Can you work these out from the model? Positions are in its coordinate system, mm. Face numbers are marked on the shaded views. Coordinates: 2 decimals unless noted, no trailing zeros. Loops run counter-clockwise (first coordinate to the right, second up) from the corner with the lowest first, then second, coordinate; pieces in that order, holes last.
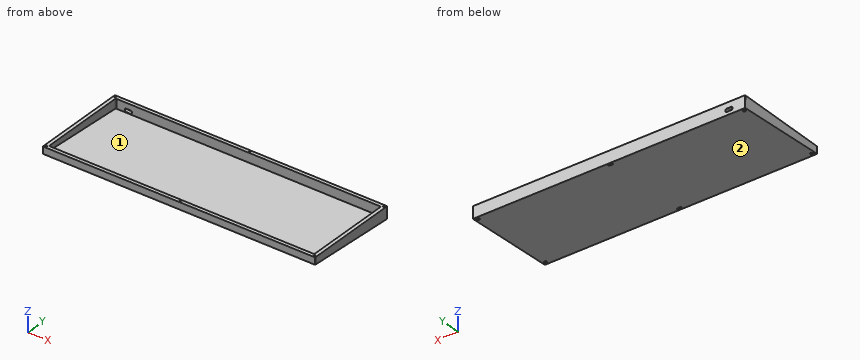
```python
from build123d import *

# Parameters (mm, degrees)
SKETCH3_W               = 431.8
SKETCH3_H               = 150.876
BOSS_EXTRUDE2_DEPTH     = 19.05
CUT_EXTRUDE4_DEPTH      = 432.8
SKETCH3_25_W            = 197.6453584
SKETCH3_25_H            = 139.766716802
SKETCH3_25_W_2          = 25.4
SKETCH3_25_W_3          = 197.645358401
CUT_EXTRUDE5_DEPTH      = 20.05
CUT_EXTRUDE5_DEPTH_BACK = 1
BOSS_EXTRUDE3_REACH     = 433.8
M2_CLEARANCE_HOLE1_D    = 2.4
CUT_EXTRUDE8_DEPTH      = 10.16
CUT_EXTRUDE9_DEPTH      = 2.032
FILLET7_R               = 1.5875
FILLET8_R               = 0.508
CUT_EXTRUDE10_REACH     = 152.876


with BuildPart() as part:
    # Sketch3 → Boss-Extrude2 (new body)
    with BuildSketch(Plane.XY):
        with Locations((169.861119801, 72.517452108)):
            Rectangle(SKETCH3_W, SKETCH3_H)
    extrude(amount=BOSS_EXTRUDE2_DEPTH)

    # Sketch11 → Cut-Extrude4 (cut, through all)
    with BuildSketch(Plane.ZY.offset(46.038880199)):
        Polygon((7.907076107, -2.920547892), (0, 147.955452108), (0, -2.920547892), align=None)
    extrude(amount=-CUT_EXTRUDE4_DEPTH, mode=Mode.SUBTRACT)

    # Sketch3<25> → Cut-Extrude5 (cut, two sides)
    with BuildSketch(Plane.XY) as cut_extrude5_sk:
        with Locations((281.383799001, 72.517452108)):
            Rectangle(SKETCH3_25_W, SKETCH3_25_H)
        with Locations((169.861119801, 72.517452108)):
            Rectangle(SKETCH3_25_W_2, SKETCH3_25_H)
        with Locations((58.338440601, 72.517452108)):
            Rectangle(SKETCH3_25_W_3, SKETCH3_25_H)
        with BuildLine():
            Line((-38.844861429, 142.400810509), (-40.4842386, 142.400810509))
            Line((-40.4842386, 142.400810509), (-40.4842386, 140.761433338))
            ThreePointArc((-40.4842386, 140.761433338), (-39.407803363, 141.324375272), (-38.844861429, 142.400810509))
        make_face()
        with BuildLine():
            ThreePointArc((-38.844861429, 2.634093707), (-39.407803363, 3.710528944), (-40.4842386, 4.273470879))
            Line((-40.4842386, 4.273470879), (-40.4842386, 2.634093707))
            Line((-40.4842386, 2.634093707), (-38.844861429, 2.634093707))
        make_face()
        with BuildLine():
            ThreePointArc((380.206478201, 4.273470879), (379.130042964, 3.710528944), (378.56710103, 2.634093707))
            Line((378.56710103, 2.634093707), (380.206478201, 2.634093707))
            Line((380.206478201, 2.634093707), (380.206478201, 4.273470879))
        make_face()
        with BuildLine():
            Line((380.206478201, 142.400810509), (378.56710103, 142.400810509))
            ThreePointArc((378.56710103, 142.400810509), (379.130042964, 141.324375272), (380.206478201, 140.761433338))
            Line((380.206478201, 140.761433338), (380.206478201, 142.400810509))
        make_face()
    extrude(amount=CUT_EXTRUDE5_DEPTH, mode=Mode.SUBTRACT)
    extrude(cut_extrude5_sk.sketch, amount=-CUT_EXTRUDE5_DEPTH_BACK, mode=Mode.SUBTRACT)

    # Sketch11<3> → Boss-Extrude3 (add, up to next)
    with BuildSketch(Plane.ZY.offset(46.038880199), mode=Mode.PRIVATE) as boss_extrude3_sk1:
        Polygon((3.815228638, 147.955452108), (0, 147.955452108), (7.907076107, -2.920547892), (11.722304745, -2.920547892), align=None)
    boss_extrude3_tool1 = extrude(boss_extrude3_sk1.sketch, amount=-BOSS_EXTRUDE3_REACH, mode=Mode.PRIVATE) - part.part
    add(boss_extrude3_tool1.solids().sort_by_distance((-46.03888, 72.517452, 5.861152))[0])

    # M2 Clearance Hole1 (through all)
    with Locations(Plane.XY.offset(19.05)):
        with Locations((-42.863880199, 144.780452108), (169.861119801, 144.780452108), (382.586119801, 144.780452108), (382.586119801, 0.254452108), (169.861119801, 0.254452108), (-42.863880199, 0.254452108)):
            Hole(M2_CLEARANCE_HOLE1_D / 2)

    # Sketch3<27> → Cut-Extrude8 (cut)
    with BuildSketch(Plane.XY):
        with BuildLine():
            Line((-44.795957036, 1.196057231), (-42.281485322, 3.710528944))
            ThreePointArc((-42.281485322, 3.710528944), (-39.407803363, 3.710528944), (-39.407803363, 0.836846986))
            Line((-39.407803363, 0.836846986), (-41.922275077, -1.677624728))
            ThreePointArc((-41.922275077, -1.677624728), (-44.795957036, -1.677624728), (-44.795957036, 1.196057231))
        make_face()
        with BuildLine():
            Line((168.083119801, 2.286452108), (171.639119801, 2.286452108))
            ThreePointArc((171.639119801, 2.286452108), (173.671119801, 0.254452108), (171.639119801, -1.777547892))
            Line((171.639119801, -1.777547892), (168.083119801, -1.777547892))
            ThreePointArc((168.083119801, -1.777547892), (166.051119801, 0.254452108), (168.083119801, 2.286452108))
        make_face()
        with BuildLine():
            Line((382.003724923, 3.710528944), (384.518196637, 1.196057231))
            ThreePointArc((384.518196637, 1.196057231), (384.518196637, -1.677624728), (381.644514678, -1.677624728))
            Line((381.644514678, -1.677624728), (379.130042964, 0.836846986))
            ThreePointArc((379.130042964, 0.836846986), (379.130042964, 3.710528944), (382.003724923, 3.710528944))
        make_face()
    extrude(amount=CUT_EXTRUDE8_DEPTH, mode=Mode.SUBTRACT)

    # Sketch3<28> → Cut-Extrude9 (cut)
    with BuildSketch(Plane.XY):
        with BuildLine():
            Line((168.083119801, 142.748452108), (171.639119801, 142.748452108))
            ThreePointArc((171.639119801, 142.748452108), (173.671119801, 144.780452108), (171.639119801, 146.812452108))
            Line((171.639119801, 146.812452108), (168.083119801, 146.812452108))
            ThreePointArc((168.083119801, 146.812452108), (166.051119801, 144.780452108), (168.083119801, 142.748452108))
        make_face()
        with BuildLine():
            Line((379.130042964, 144.198057231), (381.644514678, 146.712528944))
            ThreePointArc((381.644514678, 146.712528944), (384.518196637, 146.712528944), (384.518196637, 143.838846986))
            Line((384.518196637, 143.838846986), (382.003724923, 141.324375272))
            ThreePointArc((382.003724923, 141.324375272), (379.130042964, 141.324375272), (379.130042964, 144.198057231))
        make_face()
        with BuildLine():
            Line((-44.795957036, 143.838846986), (-42.281485322, 141.324375272))
            ThreePointArc((-42.281485322, 141.324375272), (-39.407803363, 141.324375272), (-39.407803363, 144.198057231))
            Line((-39.407803363, 144.198057231), (-41.922275077, 146.712528944))
            ThreePointArc((-41.922275077, 146.712528944), (-44.795957036, 146.712528944), (-44.795957036, 143.838846986))
        make_face()
    extrude(amount=CUT_EXTRUDE9_DEPTH, mode=Mode.SUBTRACT)

    # Fillet7
    fillet7_edges = [part.edges().sort_by_distance(p)[0] for p in [
        (380.206478201, 2.634093707, 15.240599157),
        (380.206478201, 142.400810509, 11.578167535),
        (-40.4842386, 142.400810509, 11.578167535),
        (-40.4842386, 2.634093707, 15.240599157),
    ]]
    fillet(fillet7_edges, radius=FILLET7_R)

    # Fillet8
    fillet8_edges = [part.edges().sort_by_distance(p)[0] for p in [
        (385.761119801, 147.955452108, 9.525),
        (-46.038880199, 147.955452108, 9.525),
        (-46.038880199, -2.920547892, 13.478538054),
        (385.761119801, -2.920547892, 13.478538054),
    ]]
    fillet(fillet8_edges, radius=FILLET8_R)

    # Sketch18 → Cut-Extrude10 (cut, up to next)
    with BuildSketch(Plane(origin=(0, 147.955452108, 0), x_dir=(1, 0, 0), z_dir=(0, 1, 0)), mode=Mode.PRIVATE) as cut_extrude10_sk1:
        with BuildLine():
            Line((-16.828880199, -10.16), (-23.940880199, -10.16))
            ThreePointArc((-23.940880199, -10.16), (-25.287918618, -9.602038418), (-25.845880199, -8.255))
            Line((-25.845880199, -8.255), (-25.845880199, -6.985))
            ThreePointArc((-25.845880199, -6.985), (-25.287918618, -5.637961582), (-23.940880199, -5.08))
            Line((-23.940880199, -5.08), (-16.828880199, -5.08))
            ThreePointArc((-16.828880199, -5.08), (-15.481841781, -5.637961582), (-14.923880199, -6.985))
            Line((-14.923880199, -6.985), (-14.923880199, -8.255))
            ThreePointArc((-14.923880199, -8.255), (-15.481841781, -9.602038418), (-16.828880199, -10.16))
        make_face()
    cut_extrude10_tool1 = extrude(cut_extrude10_sk1.sketch, amount=-CUT_EXTRUDE10_REACH, mode=Mode.PRIVATE) & part.part
    add(cut_extrude10_tool1.solids().sort_by_distance((-20.38488, 147.955452, 7.62))[0], mode=Mode.SUBTRACT)


solid = part.part
```
(1) If I drill on probe 1 along X at (y, z) = (106, 12.5); probe 2 along Y at (x, z) = (339.5, 12.5); probe 3 along Z at (x, y) = (-12, 62), over which ranges is the centre line in solid material (lowest first)?
Check values:
probe 1: x = -46.04 to -40.48, 380.21 to 385.76
probe 2: y = -2.92 to 2.63, 142.4 to 147.96
probe 3: z = 4.5 to 8.32
(2) I want a section at A-A on x = 234.5. Write out the boundary of the cut face in (y, z), then the cut area to 3 significant figures.
Check values:
outline: (-2.92, 7.91) - (147.96, 0) - (147.96, 19.05) - (142.4, 19.05) - (142.4, 4.11) - (2.63, 11.43) - (2.63, 19.05) - (-2.92, 19.05) - close
area: 701 mm2
(3) I'm going to push flat-ended pins straight in: pin 1 (7 mm diameter, centred on x = 382.5, y = -0.5, fed in from -Z); pin 2 (8 mm diameter, centred on x = 54.5, y = 115.5, fed in from -Z); pin 3 (3 mm diameter, centred on x = 382.59, y = 0.25, fed in from -Z); pin 4 (1.9 mm diameter, centred on x = 169.86, y = 144.78, fed in from +Z). Where does each tip first touch, or does it pass through?
Check values:
pin 1: stops at z = 7.6
pin 2: stops at z = 1.49
pin 3: stops at z = 10.16
pin 4: passes through
(4) I want a section at B-B on y = 115. Write out the boundary of the cut face in (x, z), then the cut area to 3 significant figures.
Check values:
outline: (-46.04, 1.73) - (385.76, 1.73) - (385.76, 19.05) - (380.21, 19.05) - (380.21, 5.54) - (-40.48, 5.54) - (-40.48, 19.05) - (-46.04, 19.05) - close
area: 1,800 mm2
(5) If we mould it in two halves opening along Y, with no side actions, what happens to the marked faces 1 and 2? For each: released by +Y, released by -Y, zero draft, split by the parting line, or undercut.
Check values:
face 1: undercut
face 2: released by -Y
